Input: part model. Units: mm. Frame: model coordinates. Face numbers are marked on the shaded views. Round coordinates to 2 decimals unless told otherwise and drop trailing zeros. Order: outer loops, then holes, each group sorted by start corner. A loop starts at its lowest first (then second) coordinate and runs counter-clockwise, first axis right, second up. Notation, with made-up numbers: (81.5, 18) -> (104.5, 18) arc R22 ccw to (104.5, 24) -> close; hole circle Ø1 at (24, 36.25). An arc over 180 degrees is marked (long way). Use a Markdown table: item, result.
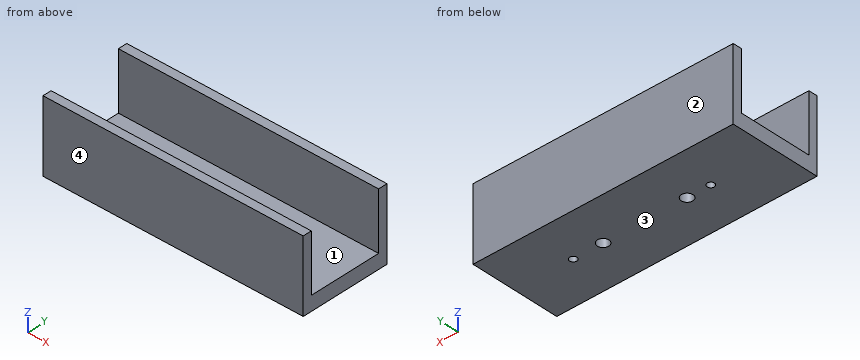
Autodesk Fusion 360 part; units mm, degrees
sketch "Sketch1" plane through (0, 0, 0) normal (0, 0, 1) x (1, 0, 0) in component "Mount"
  line L0 (0, 0) -> (89.85, 0)
  line L1 (89.85, 0) -> (89.85, 31.11)
  line L2 (89.85, 31.11) -> (0, 31.11)
  line L3 (0, 31.11) -> (0, 0)
  dimension "d1" = 89.85
  dimension "d2" = 31.11
extrude "Extrude1" add sketch "Sketch1" along normal blind 5 in component "Mount"
sketch "Sketch2" plane through (0, 0, 5) normal (0, 0, 1) x (-1, 0, 0) in component "Mount"
  line L0 (0, -31.11) -> (0, 0)
  line L1 (0, 0) -> (-89.85, 0)
  line L2 (-89.85, 0) -> (-89.85, -31.11)
  line L3 (-89.85, -31.11) -> (0, -31.11)
  line L4 (-44.925, -31.11) -> (-44.925, -28.11) construction
  line L5 (-44.925, 0) -> (-44.925, -3) construction
  line L6 (0, -3) -> (-89.85, -3)
  line L7 (0, -28) -> (-89.85, -28)
  dimension "d5" = 3
  dimension "d6" = 3
extrude "Extrude2" add sketch "Sketch2" along normal blind 20 contours L0 L2 L3 L7 | L0 L1 L2 L6 in component "Mount"
sketch "Sketch3" plane through (0, 0, 5) normal (0, 0, 1) x (-1, 0, 0) in component "Mount"
  line L0 (0, -3) -> (-89.85, -3)
  line L1 (-89.85, -3) -> (-89.85, -28)
  line L2 (-89.85, -28) -> (0, -28)
  line L3 (0, -28) -> (0, -3)
  line L4 (-44.925, -28) -> (-44.925, -3) construction
  line L5 (-89.85, -15.5) -> (0, -15.5) construction
  line L6 (-44.925, -15.5) -> (-63.425, -15.5) construction
  line L7 (-44.925, -15.5) -> (-26.425, -15.5) construction
  line L8 (-63.425, -15.5) -> (-59.425, -15.5) construction
  line L9 (-26.425, -15.5) -> (-30.425, -15.5) construction
  circle A0 centre (-30.425, -15.5) radius 4 construction
  circle A1 centre (-59.425, -15.5) radius 4 construction
  line L10 (0, -15.5) -> (-21, -15.5) construction
  line L11 (-21, -15.5) -> (-22.25, -15.5) construction
  circle A2 centre (-22.25, -15.5) radius 1.25
  line L12 (-23.5, -15.5) -> (-68.5, -15.5) construction
  line L13 (-68.5, -15.5) -> (-69.75, -15.5) construction
  circle A3 centre (-69.75, -15.5) radius 1.25
  circle A4 centre (-30.425, -15.5) radius 2
  circle A5 centre (-59.425, -15.5) radius 2
  dimension "d9" = 18.5
  dimension "d10" = 18.5
  dimension "d11" = 4
  dimension "d12" = 4
  dimension "d13" = 8
  dimension "d14" = 8
  dimension "d15" = 21
  dimension "d16" = 1.25
  dimension "d17" = 2.5
  dimension "d18" = 45
  dimension "d19" = 1.25
  dimension "d20" = 2.5
  dimension "d21" = 4
  dimension "d22" = 4
extrude "Extrude3" cut sketch "Sketch3" against normal blind 5 contours A2 | A3 | A4 | A5 in component "Mount"
component "Mount" placed x (1, 0, 0) y (0, 1, 0) z (0, 0, 1) at (0, 0, 0)
1) Pin query (flat end, axial travel): pin 1 Ø3 at (x, y) = (69.75, 15.5) entering from +Z; pin 2 Ø10 at (x, z) = (47, 14) entering from -Y. Return the tip coordinate at first contact, or that it passes through.
Results found:
| item | result |
|---|---|
| pin 1 | stops at z = 5 |
| pin 2 | stops at y = 0 |
2) Line query: L1, parallel to X at y = 15.5, z = 2.3 (3 decimals); L2, parallel to Y at x = 69, z = 20.75; L3, parallel to Y at x = 69.75, z = 2.45. Output: solid intervals per line, ascending. Write a range as [from, to].
Results found:
| item | result |
|---|---|
| L1 | x = [0, 21], [23.5, 28.425], [32.425, 57.425], [61.425, 68.5], [71, 89.85] |
| L2 | y = [0, 3], [28, 31.11] |
| L3 | y = [0, 14.25], [16.75, 31.11] |
3) Cut plane A-A on z = 11.75. Return loops of the section in (x, y).
Results found:
| item | result |
|---|---|
| outline | (0, 0) -> (89.85, 0) -> (89.85, 3) -> (0, 3) -> close; (0, 28) -> (89.85, 28) -> (89.85, 31.11) -> (0, 31.11) -> close |
4) Cut plane D-D on x = 36. Return loops of the section in (y, z).
Results found:
| item | result |
|---|---|
| outline | (0, 0) -> (31.11, 0) -> (31.11, 25) -> (28, 25) -> (28, 5) -> (3, 5) -> (3, 25) -> (0, 25) -> close |
5) Cut plane B-B on y = 15.5. Return loops of the section in (x, z) (3 decimals), and give its area (3 significant figures).
Results found:
| item | result |
|---|---|
| outline | (0, 0) -> (21, 0) -> (21, 5) -> (0, 5) -> close; (23.5, 0) -> (28.425, 0) -> (28.425, 5) -> (23.5, 5) -> close; (32.425, 0) -> (57.425, 0) -> (57.425, 5) -> (32.425, 5) -> close; (61.425, 0) -> (68.5, 0) -> (68.5, 5) -> (61.425, 5) -> close; (71, 0) -> (89.85, 0) -> (89.85, 5) -> (71, 5) -> close |
| area | 384 mm² |
6) Cut plane C-C on x = 69.75. Return loops of the section in (y, z), and give its area (3 significant figures).
Results found:
| item | result |
|---|---|
| outline | (0, 0) -> (14.25, 0) -> (14.25, 5) -> (3, 5) -> (3, 25) -> (0, 25) -> close; (16.75, 0) -> (31.11, 0) -> (31.11, 25) -> (28, 25) -> (28, 5) -> (16.75, 5) -> close |
| area | 265 mm² |
7) Pull-direction query (Y, two-part tool) for the marked faces 1, 2, 3 and 4; classes: +Y half, -Y half, draft (parallel to the pull), parting line (faces both ways), or undercut.
Results found:
| item | result |
|---|---|
| face 1 | undercut |
| face 2 | +Y half |
| face 3 | draft |
| face 4 | -Y half |
